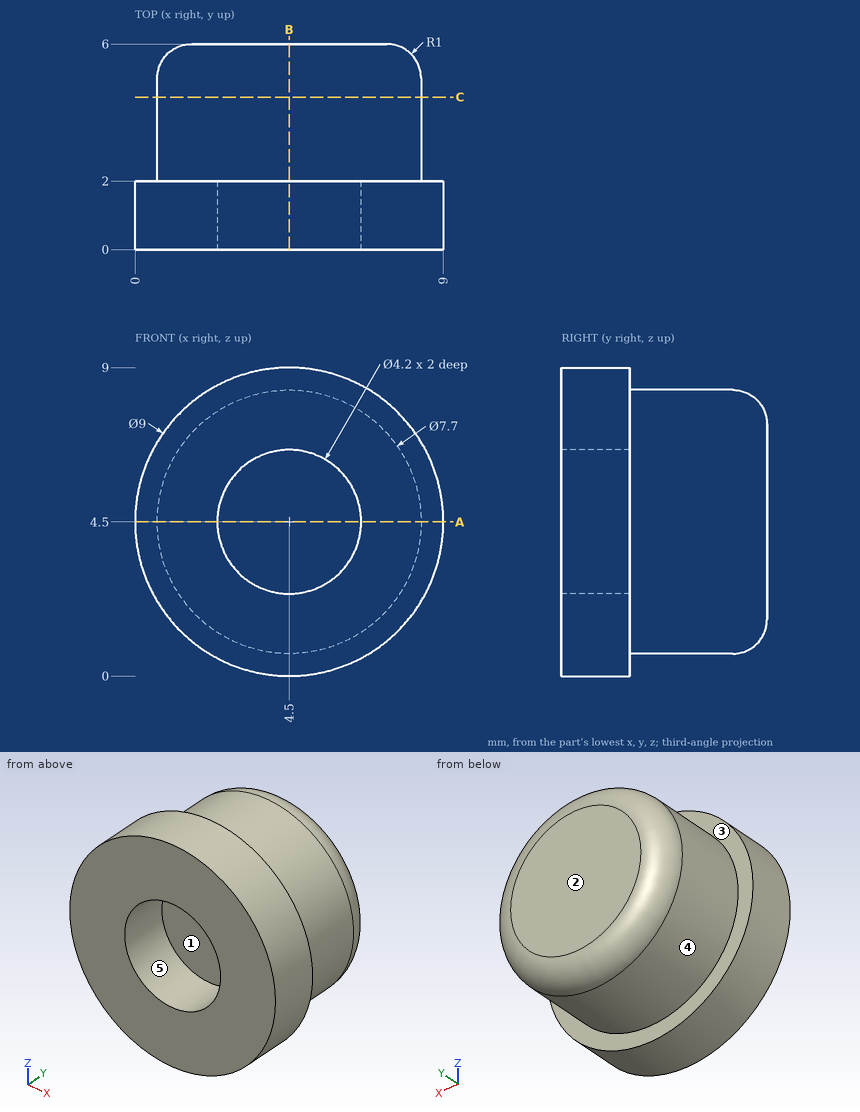
Could you check a few things on this drawing? It's one solid part, dimensions in mm from its lowest x, y, z. A direction names the side the tool comes from. Give positions to 0.01 mm unless a question says otherwise; leave off trailing zeros. Order: outer loops, then holes, each group sorted by start corner. A loop starts at its lowest first (then second) coordinate and runs counter-clockwise, first axis right, second up. Notation, with made-up numbers: (15.25, 89) - (39.25, 89) arc R23 ccw to (39.25, 100) - close; hole circle Ø5 at (-23.75, 70). An arc over 180 degrees is marked (long way). Return JSON: item names as keys, results as strings. Group by question number.
Q1. Thinking about a two-plate mould opening in Z: for the marked faces 3, 4 and 5, which applies, pulls with the +Z half, pulls with the -Z half, needs draft (parallel to the pull), parting line crosses it, or undercut?
Q2. Suppose I cut it at A-A, the plane z = 4.5. Please give me the cut outline in (x, y).
Q3. Please list where these lines run through material, in increasing order: line 1 along Z through (x, y) = (4.5, 0.7); line 2 along Y through (x, z) = (7.5, 7.5); line 3 along Y through (x, z) = (2.5, 4.5). Write a range as [from, to].
Q4. Suppose I cut it at B-B, the plane x = 4.5. Please give me the cut outline in (y, z).
Q5. Suppose I cut it at C-C, the plane y = 4.45. Please give me the cut outline in (x, z), and give its area (3 significant figures).
Q6. Which directions (+Z, -Z, +X, -X, +Y, -Y) give clear straight access to the entire face, cutting with the end or side of a thin tool? Please do the marked faces 1 and 2.
Q7. Will these pins go through, and if not, where does the flat tip stop? pin 1 Ø2 at (y, z) = (5.5, 1) entering from +X; pin 2 Ø1 at (y, z) = (3.5, 7) entering from +X.
Resolved:
{
 "1": {"face 3": "needs draft", "face 4": "parting line crosses it", "face 5": "undercut"},
 "2": {"outline": "(0, 0) - (2.4, 0) - (2.4, 2) - (6.6, 2) - (6.6, 0) - (9, 0) - (9, 2) - (8.35, 2) - (8.35, 5) arc R1 ccw to (7.35, 6) - (1.65, 6) arc R1 ccw to (0.65, 5) - (0.65, 2) - (0, 2) - close"},
 "3": {"line 1": "z = [0, 2.4], [6.6, 9]", "line 2": "y = [0, 2]", "line 3": "y = [2, 6]"},
 "4": {"outline": "(0, 0) - (2, 0) - (2, 0.65) - (5, 0.65) arc R1 ccw to (6, 1.65) - (6, 7.35) arc R1 ccw to (5, 8.35) - (2, 8.35) - (2, 9) - (0, 9) - (0, 6.6) - (2, 6.6) - (2, 2.4) - (0, 2.4) - close"},
 "5": {"outline": "circle Ø7.7 at (4.5, 4.5)", "area": "46.6 mm2"},
 "6": {"face 1": "-Y", "face 2": "+Z, -Z, +X, -X, +Y"},
 "7": {"pin 1": "stops at x = 7.36", "pin 2": "stops at x = 7.79"}
}
